Design review of the part built by this model. Coordinates are the model's own, in mm. A direction names the side the tool comes from. Give positions to 0.01 mm unless a question says otherwise; leave off trailing zeros. Order: outer loops, then holes, each group sorted by start corner. A loop starts at its lowest first (then second) coordinate and runs counter-clockwise, first axis right, second up. Notation, with made-up numbers: M 50.5,55 L 57.5,55 A6 ccw 57.5,62 Z; hole C 52,7 d4. An arc over 180 degrees is marked long. Answer as a JSON object with one key per item and string values.
from build123d import *

# Parameters (mm, degrees)
SKETCH1_R           = 1.25
BOSS_EXTRUDE1_DEPTH = 3
SKETCH2_W           = 3
SKETCH2_H           = 40.2
BOSS_EXTRUDE2_DEPTH = 5
SKETCH4_W           = 40.2
SKETCH4_H           = 5
BOSS_EXTRUDE3_DEPTH = 8
SKETCH7_W           = 40.2
SKETCH7_H           = 5
BOSS_EXTRUDE4_DEPTH = 8
SKETCH9_R           = 1.25
CUT_EXTRUDE1_DEPTH  = 8


with BuildPart() as part:
    # Sketch1 → Boss-Extrude1 (new body)
    # profile 1 of 2: a face of its own
    with BuildSketch(Plane(origin=(0, 0, 0), x_dir=(0, 0, -1), z_dir=(1, 0, 0))):
        with BuildLine():
            Line((10.5, -40), (10.5, 0))
            ThreePointArc((10.5, 0), (-2.221347256, -10.262339712), (-9.560117404, 4.342137172))
            Line((-9.560117404, 4.342137172), (-29.7, -40))
            Line((-29.7, -40), (10.5, -40))
        make_face()
    # profile 2 of 2: a face of its own
    with BuildSketch(Plane(origin=(0, 0, 0), x_dir=(0, 0, -1), z_dir=(1, 0, 0))):
        with BuildLine():
            ThreePointArc((-9.560117404, 4.342137172), (-2.221347256, -10.262339712), (10.5, 0))
            ThreePointArc((10.5, 0), (2.221347256, 10.262339712), (-9.560117404, 4.342137172))
        make_face()
        with Locations((-7.5, -3.5)):
            Circle(SKETCH1_R, mode=Mode.SUBTRACT)
        with Locations((-3.5, -7.5)):
            Circle(SKETCH1_R, mode=Mode.SUBTRACT)
        with Locations((0, -7.5)):
            Circle(SKETCH1_R, mode=Mode.SUBTRACT)
        with Locations((3.5, -7.5)):
            Circle(SKETCH1_R, mode=Mode.SUBTRACT)
        with Locations((7.5, -3.5)):
            Circle(SKETCH1_R, mode=Mode.SUBTRACT)
        with Locations((-7.5, 0)):
            Circle(SKETCH1_R, mode=Mode.SUBTRACT)
        with Locations((-7.428270452, 3.499264905)):
            Circle(SKETCH1_R, mode=Mode.SUBTRACT)
        with Locations((-3.5, 7.5)):
            Circle(SKETCH1_R, mode=Mode.SUBTRACT)
        with Locations((0, 7.5)):
            Circle(SKETCH1_R, mode=Mode.SUBTRACT)
        with Locations((7.5, 0)):
            Circle(SKETCH1_R, mode=Mode.SUBTRACT)
        with Locations((7.5, 3.5)):
            Circle(SKETCH1_R, mode=Mode.SUBTRACT)
        with Locations((3.5, 7.5)):
            Circle(SKETCH1_R, mode=Mode.SUBTRACT)
    extrude(amount=BOSS_EXTRUDE1_DEPTH)

    # Sketch2 → Boss-Extrude2 (add)
    with BuildSketch(Plane(origin=(0, -40, 0), x_dir=(-1, 0, 0), z_dir=(0, -1, 0))):
        with Locations((-1.5, -9.6)):
            Rectangle(SKETCH2_W, SKETCH2_H)
    extrude(amount=BOSS_EXTRUDE2_DEPTH)

    # Sketch4 → Boss-Extrude3 (add)
    with BuildSketch(Plane.ZY):
        with Locations((9.6, -42.5)):
            Rectangle(SKETCH4_W, SKETCH4_H)
    extrude(amount=BOSS_EXTRUDE3_DEPTH)


with BuildPart() as body_2:
    # Mirror1: mirrored copy
    add(part.part.mirror(Plane(origin=(3, 0, 0), x_dir=(0, 0, 1), z_dir=(1, 0, 0))))

    # Sketch7 → Boss-Extrude4 (add)
    with BuildSketch(Plane.ZY.offset(-3)):
        with Locations((9.6, -42.5)):
            Rectangle(SKETCH7_W, SKETCH7_H)
    extrude(amount=BOSS_EXTRUDE4_DEPTH)

    # Sketch9 → Cut-Extrude1 (cut)
    with BuildSketch(Plane(origin=(0, -40, 0), x_dir=(1, 0, 0), z_dir=(0, 1, 0))):
        with Locations(Location((-1, 0.5, 0), (0, 0, 270))):
            Circle(SKETCH9_R)
        with Locations(Location((-1, -19.7, 0), (0, 0, 270))):
            Circle(SKETCH9_R)
    extrude(amount=-CUT_EXTRUDE1_DEPTH, mode=Mode.SUBTRACT)


solid = body_2.part
(1) We need section B-B (z = 7.5). Write out the cut boundary in (x, y), plus the area to 3 significant figures.
Checked values:
{"outline": "M -5,-45 L 14,-45 L 14,-40 L 6,-40 L 6,-4.75 L 3,-4.75 L 3,-40 L -5,-40 Z; M 3,-2.25 L 6,-2.25 L 6,-1.25 L 3,-1.25 Z; M 3,1.25 L 6,1.25 L 6,2.25 L 3,2.25 Z; M 3,4.75 L 6,4.75 L 6,7.35 L 3,7.35 Z", "area": "215 mm^2"}
(2) Tool access review of faces 5 (the flat face through (6, -20, 5)), 6 (the flat face through (3, -20, 5)), 7 (the cylindrical face through (4.52, -8.72, 0.27)): name each direction out of +Z, -Z, +X, -X, +Y, -Y from which nothing blocks a thin tool from reaching the whole face with its end or side.
Checked values:
{"face 5": "+Z, -Z, +X, +Y", "face 6": "+Z, -Z, -X, +Y", "face 7": "+X, -X"}
(3) To check wall thickness, follow L1, parallel to Y at x = 5.45, z = 0; L2, parallel to X at y = -43.7, z = -0.5; L3, parallel to X at y = -38, z = -6. State the ranges of each line that lie inside material, in increasing order. Write a range as from..to.
Checked values:
{"L1": "y = -45..-8.75, -6.25..6.25, 8.75..10.5", "L2": "x = -5..-2.25, 0.25..14", "L3": "x = 3..6"}
(4) We need section D-D (z = -4). Write out the cut boundary in (x, y).
Checked values:
{"outline": "M -5,-45 L 14,-45 L 14,-40 L 6,-40 L 6,-8.65 L 3,-8.65 L 3,-40 L -5,-40 Z; M 3,-6.35 L 6,-6.35 L 6,6.35 L 3,6.35 Z; M 3,8.65 L 6,8.65 L 6,9.71 L 3,9.71 Z"}
(5) We need section C-C (y = 7.5). Write out the cut boundary in (x, z).
Checked values:
{"outline": "M 3,-7.35 L 6,-7.35 L 6,-4.75 L 3,-4.75 Z; M 3,-2.25 L 6,-2.25 L 6,-1.25 L 3,-1.25 Z; M 3,1.25 L 6,1.25 L 6,2.25 L 3,2.25 Z; M 3,4.75 L 6,4.75 L 6,7.35 L 3,7.35 Z"}
(6) Draft analysis for pull direction Y (two halves, no side actions). For faces 1 (the cylindrical face through (4.52, -4.26, 8.49)), 2 (the flat face through (14, -42, 9)), 3 (the flat face through (-1, -40, 9)), 4 (the cylindrical face through (4.521, 7.021, -4.655)), state which applies: +Y half, -Y half, draft (parallel to the pull), parting line (faces both ways), or undercut.
Checked values:
{"face 1": "undercut", "face 2": "draft", "face 3": "+Y half", "face 4": "undercut"}
(7) Insertion check: pin 1 (3 mm diameter, centred on y = -7.5, z = -3.5, fed in from +X); pin 2 (4 mm diameter, centred on x = -1.5, z = 4, fed in from +Y); pin 3 (10 mm diameter, centred on y = -27, z = 9, fed in from -X). Each pin has a flat end and moves straight along its axis. Give the tip position at first contact, or say it passes through.
Checked values:
{"pin 1": "stops at x = 6", "pin 2": "stops at y = -40", "pin 3": "stops at x = 3"}
(8) We need section A-A (x = -1). Write out the cut boundary in (y, z).
Checked values:
{"outline": "M -45,-10.5 L -40,-10.5 L -40,-1.75 L -45,-1.75 Z; M -45,0.75 L -40,0.75 L -40,18.45 L -45,18.45 Z; M -45,20.95 L -40,20.95 L -40,29.7 L -45,29.7 Z"}
